Here's how the part is built. I have some questions about the finished solid (model axes, mm). A direction names the side the tool comes from. Round coordinates to 2 decimals unless told otherwise and drop trailing zeros. Order: outer loops, then holes, each group sorted by start corner. A loop starts at its lowest first (then second) coordinate and runs counter-clockwise, first axis right, second up. Notation, with made-up numbers: (59.5, -5.5) -> (88.5, -5.5) arc R29 ccw to (88.5, 21.5) -> close; hole circle Ø8 at (89.25, 50). An arc over 180 degrees is marked (long way). Answer in a Markdown table with one row per item.
```python
from build123d import *

# Parameters (mm, degrees)
SKETCH1_R               = 88.9
SKETCH1_R_2             = 69.85
BOSS_EXTRUDE1_DEPTH     = 17.4625
SKETCH2_R               = 69.85
BOSS_EXTRUDE2_DEPTH     = 1.5875
SKETCH3_R               = 69.85
SKETCH3_R_2             = 57.15
BOSS_EXTRUDE3_DEPTH     = 17.4625
SKETCH4_R               = 10.715625
BOSS_EXTRUDE4_DEPTH     = 7.9375
SKETCH5_R               = 9.525
BOSS_EXTRUDE5_DEPTH     = 25.4
CUT_EXTRUDE1_DEPTH      = 129.263712717
CUT_EXTRUDE1_DEPTH_BACK = 129.263712717
SKETCH6_R               = 6.35


with BuildPart() as part:
    # Sketch1 → Boss-Extrude1 (new, symmetric)
    with BuildSketch(Plane.XY):
        Circle(SKETCH1_R)
        Circle(SKETCH1_R_2, mode=Mode.SUBTRACT)
    extrude(amount=BOSS_EXTRUDE1_DEPTH, both=True)

    # Sketch2 → Boss-Extrude2 (add, symmetric)
    with BuildSketch(Plane.XY):
        Circle(SKETCH2_R)
    extrude(amount=BOSS_EXTRUDE2_DEPTH, both=True)



with BuildPart() as body_2:
    # Sketch3 → Boss-Extrude3 (new, symmetric)
    with BuildSketch(Plane.XY):
        Circle(SKETCH3_R)
        Circle(SKETCH3_R_2, mode=Mode.SUBTRACT)
    extrude(amount=BOSS_EXTRUDE3_DEPTH, both=True)


with BuildPart() as part_1:
    add(part.part)

    add(body_2.part)  # Boss-Extrude4 merges body 2
    # Sketch4 → Boss-Extrude4 (add)
    with BuildSketch(Plane.XY):
        Circle(SKETCH4_R)
    extrude(amount=BOSS_EXTRUDE4_DEPTH)

    # Sketch5 → Boss-Extrude5 (add)
    with BuildSketch(Plane.XY):
        Circle(SKETCH5_R)
    extrude(amount=-BOSS_EXTRUDE5_DEPTH)

    # Sketch6 → Cut-Extrude1 (cut, two sides: drawn at the far end of the back side and taken through both)
    with BuildSketch(Plane.XY.offset(-CUT_EXTRUDE1_DEPTH_BACK)):
        Circle(SKETCH6_R)
    extrude(amount=CUT_EXTRUDE1_DEPTH + CUT_EXTRUDE1_DEPTH_BACK, mode=Mode.SUBTRACT)


solid = part_1.part
```
1. Please list where these lines run through material, in increasing order: line 1 along Y through (x, z) = (0, -9.75) (3 decimals); line 2 along Z through (x, y) = (7, -66); line 3 along Z through (x, y) = (-15.5, 50).
Numbers:
| item | result |
|---|---|
| line 1 | y = -88.9 to -57.15, -9.525 to -6.35, 6.35 to 9.525, 57.15 to 88.9 |
| line 2 | z = -17.46 to 17.46 |
| line 3 | z = -1.59 to 1.59 |
2. We'd pull the mould along X, two halves only. Please class faces 4 (the face through (-1, -12, -1.588)), 5 (the face through (84.795, 26.703, 0.244)), 6 (the face through (-1, -58, -17.462)): released by +X, released by -X, zero draft, split by the parting line, or undercut.
Numbers:
| item | result |
|---|---|
| face 4 | undercut |
| face 5 | split by the parting line |
| face 6 | zero draft |
3. For faces 1 (the face through (-1, -12, 1.588)), 2 (the face through (2, -6.2, -25.4)), 3 (the face through (-57.095, 2.513, -9.636)), which set-ups out of +Z, -Z, +X, -X, +Y, -Y let a thin tool reach every point of the face, with its end or its side?
Numbers:
| item | result |
|---|---|
| face 1 | +Z |
| face 2 | -Z, +X, -X, +Y, -Y |
| face 3 | -Z |
4. Suppose I cut it at D-D on x = -43. Write out the boundary of the cut face in (y, z).
Numbers:
| item | result |
|---|---|
| outline | (-77.81, -17.46) -> (-37.64, -17.46) -> (-37.64, -1.59) -> (37.64, -1.59) -> (37.64, -17.46) -> (77.81, -17.46) -> (77.81, 17.46) -> (37.64, 17.46) -> (37.64, 1.59) -> (-37.64, 1.59) -> (-37.64, 17.46) -> (-77.81, 17.46) -> close |
5. Suppose I cut it at C-C on z = -5.5. Write out the boundary of the cut face in (x, y) (3 decimals).
Numbers:
| item | result |
|---|---|
| outline | circle Ø177.8 at (0, 0); circle Ø19.05 at (0, 0); hole circle Ø114.3 at (0, 0); hole circle Ø12.7 at (0, 0) |
6. For pin 1 Ø1 at (x, y) = (-9.5, 10) entering from -Z; pin 2 Ø8 at (y, z) = (-36.5, 0.5) entering from -X; pin 3 Ø8 at (x, z) = (35, 12.5) entering from -Y, each with a flat end and sliding along its axis, tell me the tip position at first contact or that it passes through.
Numbers:
| item | result |
|---|---|
| pin 1 | stops at z = -1.59 |
| pin 2 | stops at x = -82.75 |
| pin 3 | stops at y = -83.32 |
